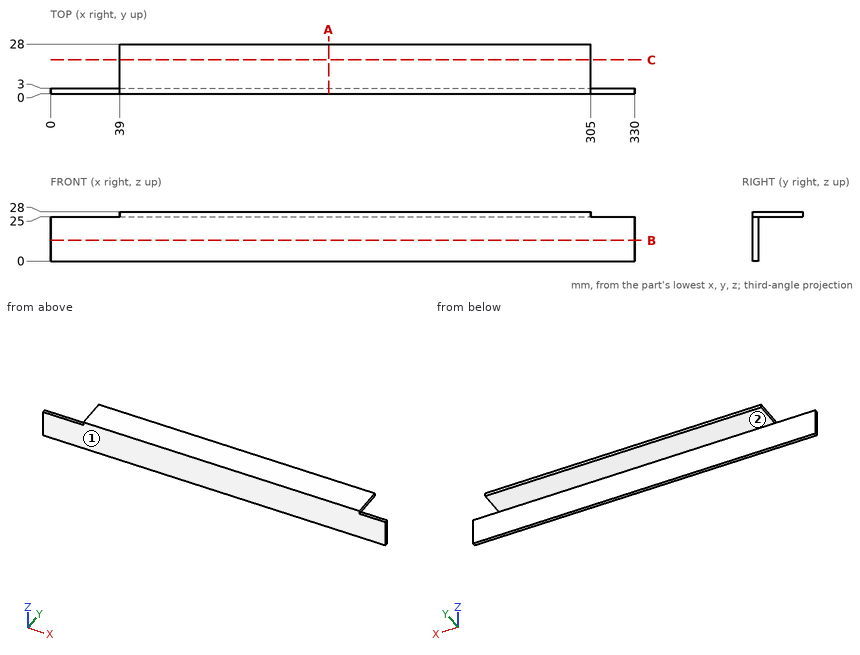
Check sheet for the drawn part. Datum: minimum x, y, z corner. Units: mm. A direction names the side the tool comes from. Coordinates: 2 decimals unless noted, no trailing zeros. Loops run counter-clockwise (first coordinate to the right, second up) from the corner with the lowest first, then second, coordinate; pieces in that order, holes last. Notation, with made-up numbers: M 88.25,-26.75 L 95.25,-26.75 A31 cw 95.25,8.25 Z; hole C -10.75,-14 d11. An arc over 180 degrees is marked long. Answer as a JSON object with one key per item and string values.
1. Scan lines: L1, parallel to Y at x = 260.5, z = 20; L2, parallel to Z at x = 41, y = 5. Record each from-to range of solid material in increasing order. Write a range as from..to.
Outcome:
{"L1": "0..3", "L2": "25..28"}
2. Sectioned sample at C-C on y = 19. Record the cut outline in (x, z).
Outcome:
{"outline": "M 39,25 L 305,25 L 305,28 L 39,28 Z"}
3. Depth check by flat-ended pin: P1, Ø0.9, axis at y = 9.5, z = 27, coming from the -X side; P2, Ø0.9, axis at x = 317, y = 1, coming from the +Z side; P3, Ø3.5, axis at y = 11.5, z = 26, coming from the +X side. Enter the tip coordinate at first touch or a pass-through.
Outcome:
{"P1": "x = 39", "P2": "z = 25", "P3": "x = 305"}
4. Sectioned sample at B-B on z = 11.75. Record the cut outline in (x, y).
Outcome:
{"outline": "M 0,0 L 330,0 L 330,3 L 0,3 Z"}
5. Access from +Z, -Z, +X, -X, +Y, -Y to the whole of each face (thin tool, end or side, straight path). Record for the marked faces 1 and 2.
Outcome:
{"face 1": "+Z, -Z, +X, -X, -Y", "face 2": "-Z, +X, -X, +Y"}
6. Sectioned sample at A-A on x = 157. Record the cut outline in (y, z), and give its area (3 significant figures).
Outcome:
{"outline": "M 0,0 L 3,0 L 3,25 L 28,25 L 28,28 L 0,28 Z", "area": "159 mm²"}
